Autodesk Inventor part; units mm, degrees
ref_plane "YZ Plane" through (0, 0, 0) normal (1, 0, 0) x (0, 1, 0)
ref_plane "XZ Plane" through (0, 0, 0) normal (0, 1, 0) x (-1, 0, 0)
ref_plane "XY Plane" through (0, 0, 0) normal (0, 0, 1) x (1, 0, 0)
sketch "Sketch1" plane through (0, 0, 0) normal (1, 0, 0) x (0, 1, 0)
  line L0 (-40.5, 30) -> (-40.5, -30)
  line L1 (-40.5, -30) -> (40.5, -30)
  line L2 (40.5, -30) -> (40.5, 30)
  line L3 (40.5, 30) -> (-40.5, 30)
  line L4 (-40.5, 30) -> (40.5, -30) construction
  line L5 (-40.5, -30) -> (40.5, 30) construction
  line L6 (-40.5, 18) -> (-40.5, 6)
  line L7 (-40.5, 6) -> (-43.5, 6)
  line L8 (-43.5, 6) -> (-43.5, 18)
  line L9 (-43.5, 18) -> (-40.5, 18)
  line L10 (-40.5, -6) -> (-40.5, -18)
  line L11 (-40.5, -18) -> (-43.5, -18)
  line L12 (-43.5, -18) -> (-43.5, -6)
  line L13 (-43.5, -6) -> (-40.5, -6)
  line L14 (-8.1, -30) -> (-8.1, -33)
  line L15 (-8.1, -33) -> (-24.3, -33)
  line L16 (-24.3, -33) -> (-24.3, -30)
  line L17 (-24.3, -30) -> (-8.1, -30)
  line L18 (8.1, -30) -> (24.3, -30)
  line L19 (24.3, -30) -> (24.3, -33)
  line L20 (24.3, -33) -> (8.1, -33)
  line L21 (8.1, -33) -> (8.1, -30)
  line L22 (-60.9, 0) -> (60.9, 0)
  line L23 (0, -45.6) -> (0, 42.6)
  line L24 (40.5, 18) -> (40.5, 6)
  line L25 (40.5, 6) -> (43.5, 6)
  line L26 (43.5, 6) -> (43.5, 18)
  line L27 (43.5, 18) -> (40.5, 18)
  line L28 (40.5, -6) -> (40.5, -18)
  line L29 (40.5, -18) -> (43.5, -18)
  line L30 (43.5, -18) -> (43.5, -6)
  line L31 (43.5, -6) -> (40.5, -6)
  point P0 (0, 0)
  point P1 (-43.5, -12)
  point P2 (43.5, -12)
  dimension "d0" = 81
  dimension "d1" = 60
  dimension "d2" = 3
  dimension "d3" = 12
  dimension "d4" = 12
  dimension "d5" = 12
  dimension "d6" = 12
  dimension "d7" = 16.2
  dimension "d8" = 16.2
  dimension "d9" = 16.2
  dimension "d10" = 16.2
extrude "Extrusion1" add sketch "Sketch1" along normal blind 3
sketch "Sketch2" plane through (3, 0, 0) normal (1, 0, 0) x (0, 0, -1)
  line L0 (-30, 40.5) -> (-30, -40.5)
  line L1 (-30, -40.5) -> (-30, 40.5)
  line L2 (-30, 40.5) -> (-33, 40.5)
  line L3 (-33, 40.5) -> (-33, -40.5)
  line L4 (-33, -40.5) -> (-30, -40.5)
  point P0 (0, 0)
  dimension "d13" = 3
extrude "Extrusion2" add sketch "Sketch2" against normal blind 3
equation "\"d3\" = 0.2 * d1"
equation "\"d4\" = d3"
equation "\"d5\" = d3"
equation "\"d6\" = d4"
equation "\"d7\" = 0.2 * d0"
equation "\"d8\" = d7"
equation "\"d9\" = d7"
equation "\"d10\" = d8"
equation "\"d13\" = d2"
equation "\"d14\" = d2"
properties part number "back"
Geometry: final body of the model. Coordinates: model frame, mm. A direction names the side the tool comes from. Give positions to 0.01 mm unless a question says otherwise; leave off trailing zeros. Write each loop counter-clockwise with the first axis right and the second up, starting at its lowest first coordinate (ties: lowest second). Pieces come first, ordered by that corner, then holes.
1. Draft query along Z for faces 6 (the flat face through (1, 42, 18)), 7 (the flat face through (1, 42, -6)), 8 (the flat face through (1, -42, -6)), 9 (the flat face through (1, 42, -18)). Return one class per face: released by +Z, released by -Z, zero draft, split by the parting line, or undercut.
2. Section query C-C, the plane y = 38. Return loops of the section in (x, z), then the cut area to 3 significant figures.
3. Section query A-A, the plane x = 1.4. Return loops of the section in (y, z).
4. Section query B-B, the plane z = -21. Return loops of the section in (x, y), then the cut area to 3 significant figures.
5. Reachability of faces 1 (the flat face through (2, 40.5, 25)), 2 (the flat face through (1, -42, 18)), 3 (the flat face through (1, -40.5, -24)), 4 (the flat face through (1, 24.3, -31)), 5 (the flat face through (1, 42, 6)) from +Z, -Z, +X, -X, +Y, -Y: full face, straight path, thin tool, end or side. Return the list, or none.
6. Pin query (flat end, axial travel): P1, Ø0.9, axis at x = 2, z = 25.5, coming from the -Y side; P2, Ø1.5, axis at x = 1, z = -32, coming from the +Y side; P3, Ø1.5, axis at x = 2, z = -26.5, coming from the +Y side. Return the tip coordinate at first contact, or that it passes through.
7. Line query: probe 1 along Y at (x, z) = (0.75, 22.5); probe 2 along Z at (x, y) = (1.45, -25). Output: solid intervals per line, ascending.
Computed:
1. face 6: released by +Z
1. face 7: undercut
1. face 8: undercut
1. face 9: released by -Z
2. outline: (0, -30) - (3, -30) - (3, 33) - (0, 33) - close
2. area: 189 mm2
3. outline: (-43.5, -18) - (-40.5, -18) - (-40.5, -30) - (-24.3, -30) - (-24.3, -33) - (-8.1, -33) - (-8.1, -30) - (8.1, -30) - (8.1, -33) - (24.3, -33) - (24.3, -30) - (40.5, -30) - (40.5, -18) - (43.5, -18) - (43.5, -6) - (40.5, -6) - (40.5, 6) - (43.5, 6) - (43.5, 18) - (40.5, 18) - (40.5, 33) - (-40.5, 33) - (-40.5, 18) - (-43.5, 18) - (-43.5, 6) - (-40.5, 6) - (-40.5, -6) - (-43.5, -6) - close
4. outline: (0, -40.5) - (3, -40.5) - (3, 40.5) - (0, 40.5) - close
4. area: 243 mm2
5. face 1: +Z, +X, -X, +Y
5. face 2: +Z, +X, -X, -Y
5. face 3: -Z, +X, -X, -Y
5. face 4: -Z, +X, -X, +Y
5. face 5: +X, -X, +Y
6. P1: stops at y = -40.5
6. P2: stops at y = 24.3
6. P3: stops at y = 40.5
7. probe 1: y = -40.5 to 40.5
7. probe 2: z = -30 to 33
